from build123d import *

# Parameters (mm, degrees)
SKETCH1_W                 = 113.5
SKETCH1_H                 = 8.5
BOSS_EXTRUDE1_DEPTH       = 8.5
BOSS_EXTRUDE2_DEPTH       = 5
BOSS_EXTRUDE3_DEPTH       = 5
SKETCH13_W                = 91.5
SKETCH13_H                = 6.5
CUT_EXTRUDE1_DEPTH        = 6.5
M3X0_5_TAPPED_HOLE1_D     = 2.5
M3X0_5_TAPPED_HOLE1_DEPTH = 7.5
M3X0_5_TAPPED_HOLE1_TIP   = 0.751075774
M3X0_5_TAPPED_HOLE2_D     = 2.5
M3X0_5_TAPPED_HOLE2_DEPTH = 5
M3X0_5_TAPPED_HOLE3_D     = 2.5
M3X0_5_TAPPED_HOLE3_DEPTH = 5
M3X0_5_TAPPED_HOLE4_D     = 2.5
M3X0_5_TAPPED_HOLE4_DEPTH = 7.5
M3X0_5_TAPPED_HOLE4_TIP   = 0.751075774
FILLET1_R                 = 1
FILLET2_R                 = 1
FILLET3_R                 = 1
FILLET4_R                 = 3
M3X0_5_TAPPED_HOLE5_D     = 2.5
M3X0_5_TAPPED_HOLE5_DEPTH = 7.5
M3X0_5_TAPPED_HOLE5_TIP   = 0.751075774
M3X0_5_TAPPED_HOLE6_D     = 2.5
M3X0_5_TAPPED_HOLE6_DEPTH = 7.5
M3X0_5_TAPPED_HOLE6_TIP   = 0.751075774
M3X0_5_TAPPED_HOLE7_D     = 2.5
M3X0_5_TAPPED_HOLE7_DEPTH = 7.5
M3X0_5_TAPPED_HOLE7_TIP   = 0.751075774
M3X0_5_TAPPED_HOLE9_D     = 2.5
M3X0_5_TAPPED_HOLE9_DEPTH = 7.5
M3X0_5_TAPPED_HOLE9_TIP   = 0.751075774
SKETCH43_W                = 10.5
SKETCH43_H                = 10.5
CUT_EXTRUDE3_DEPTH        = 110.01404726
SKETCH44_R                = 2.5
CUT_EXTRUDE4_DEPTH        = 10
CUT_EXTRUDE5_REACH        = 107.072
SKETCH45_R                = 1.25
M6_TAPPED_HOLE1_D         = 5
M6_TAPPED_HOLE1_DEPTH     = 3.05
M6_TAPPED_HOLE1_TIP       = 1.502151548


with BuildPart() as part:
    # Sketch1 → Boss-Extrude1 (new body)
    with BuildSketch(Plane.XY):
        Rectangle(SKETCH1_W, SKETCH1_H)
    extrude(amount=BOSS_EXTRUDE1_DEPTH)

    # Sketch4 → Boss-Extrude2 (add)
    with BuildSketch(Plane(origin=(50.75, 0, 0), x_dir=(0, 0, -1), z_dir=(1, 0, 0))):
        Polygon((0, -2.25), (10.5, -2.25), (10.5, 14.75), (-6.5, 14.75), (-6.5, 4.25), (0, 4.25), align=None)
    extrude(amount=-BOSS_EXTRUDE2_DEPTH)

    # Sketch12 → Boss-Extrude3 (add)
    with BuildSketch(Plane.ZY.offset(50.75)):
        Polygon((6.5, 4.25), (6.5, 14.75), (-10.5, 14.75), (-10.5, -2.25), (0, -2.25), (0, 4.25), align=None)
    extrude(amount=-BOSS_EXTRUDE3_DEPTH)

    # Sketch13 → Cut-Extrude1 (cut)
    with BuildSketch(Plane(origin=(0, 4.25, 0), x_dir=(1, 0, 0), z_dir=(0, 1, 0))):
        with Locations((0, -3.25)):
            Rectangle(SKETCH13_W, SKETCH13_H)
    extrude(amount=-CUT_EXTRUDE1_DEPTH, mode=Mode.SUBTRACT)

    # M3x0.5 Tapped Hole1
    with Locations(Plane.XY.offset(6.5)):
        with Locations((-48.25, 7.75)):
            Hole(M3X0_5_TAPPED_HOLE1_D / 2, depth=M3X0_5_TAPPED_HOLE1_DEPTH)
            with Locations((0, 0, -(M3X0_5_TAPPED_HOLE1_DEPTH + M3X0_5_TAPPED_HOLE1_TIP / 2))):  # 118° drill point
                Cone(0, M3X0_5_TAPPED_HOLE1_D / 2, M3X0_5_TAPPED_HOLE1_TIP, mode=Mode.SUBTRACT)

    # M3x0.5 Tapped Hole2
    with Locations(Plane.ZY.offset(50.75)):
        with Locations((3.25, 12.25)):
            Hole(M3X0_5_TAPPED_HOLE2_D / 2, depth=M3X0_5_TAPPED_HOLE2_DEPTH)

    # M3x0.5 Tapped Hole3
    with Locations(Plane.ZY.offset(50.75)):
        with Locations((-8, 1)):
            Hole(M3X0_5_TAPPED_HOLE3_D / 2, depth=M3X0_5_TAPPED_HOLE3_DEPTH)

    # M3x0.5 Tapped Hole4
    with Locations(Plane.XZ.offset(2.25)):
        with Locations((-48.25, -3.5)):
            Hole(M3X0_5_TAPPED_HOLE4_D / 2, depth=M3X0_5_TAPPED_HOLE4_DEPTH)
            with Locations((0, 0, -(M3X0_5_TAPPED_HOLE4_DEPTH + M3X0_5_TAPPED_HOLE4_TIP / 2))):  # 118° drill point
                Cone(0, M3X0_5_TAPPED_HOLE4_D / 2, M3X0_5_TAPPED_HOLE4_TIP, mode=Mode.SUBTRACT)

    # Fillet1
    fillet1_edges = [part.edges().sort_by_distance(p)[0] for p in [
        (0, -4.25, 8.5),
    ]]
    fillet(fillet1_edges, radius=FILLET1_R)

    # Fillet2
    fillet2_edges = [part.edges().sort_by_distance(p)[0] for p in [
        (-56.75, 0.5, 8.5),
        (-56.75, 0, 0),
        (-56.75, 4.25, 4.25),
        (-56.75, -4.25, 3.75),
        (-56.75, -3.957106781, 8.207106781),
    ]]
    fillet(fillet2_edges, radius=FILLET2_R)

    # Fillet3
    fillet3_edges = [part.edges().sort_by_distance(p)[0] for p in [
        (56.75, 0, 0),
        (56.75, 4.25, 4.25),
        (56.75, 0.5, 8.5),
        (56.75, -4.25, 3.75),
        (56.75, -3.957106781, 8.207106781),
    ]]
    fillet(fillet3_edges, radius=FILLET3_R)

    # Fillet4
    fillet4_edges = [part.edges().sort_by_distance(p)[0] for p in [
        (-45.75, 1, 6.5),
        (45.75, 1, 6.5),
    ]]
    fillet(fillet4_edges, radius=FILLET4_R)

    # M3x0.5 Tapped Hole5
    with Locations(Plane.XY.offset(6.5)):
        with Locations((48.25, 7.75)):
            Hole(M3X0_5_TAPPED_HOLE5_D / 2, depth=M3X0_5_TAPPED_HOLE5_DEPTH)
            with Locations((0, 0, -(M3X0_5_TAPPED_HOLE5_DEPTH + M3X0_5_TAPPED_HOLE5_TIP / 2))):  # 118° drill point
                Cone(0, M3X0_5_TAPPED_HOLE5_D / 2, M3X0_5_TAPPED_HOLE5_TIP, mode=Mode.SUBTRACT)

    # M3x0.5 Tapped Hole6
    with Locations(Plane.XZ.offset(2.25)):
        with Locations((48.25, -3.5)):
            Hole(M3X0_5_TAPPED_HOLE6_D / 2, depth=M3X0_5_TAPPED_HOLE6_DEPTH)
            with Locations((0, 0, -(M3X0_5_TAPPED_HOLE6_DEPTH + M3X0_5_TAPPED_HOLE6_TIP / 2))):  # 118° drill point
                Cone(0, M3X0_5_TAPPED_HOLE6_D / 2, M3X0_5_TAPPED_HOLE6_TIP, mode=Mode.SUBTRACT)

    # M3x0.5 Tapped Hole7
    with Locations(Plane(origin=(50.75, 0, 0), x_dir=(0, 0, -1), z_dir=(1, 0, 0))):
        with Locations((8, 1)):
            Hole(M3X0_5_TAPPED_HOLE7_D / 2, depth=M3X0_5_TAPPED_HOLE7_DEPTH)
            with Locations((0, 0, -(M3X0_5_TAPPED_HOLE7_DEPTH + M3X0_5_TAPPED_HOLE7_TIP / 2))):  # 118° drill point
                Cone(0, M3X0_5_TAPPED_HOLE7_D / 2, M3X0_5_TAPPED_HOLE7_TIP, mode=Mode.SUBTRACT)

    # M3x0.5 Tapped Hole9
    with Locations(Plane(origin=(50.75, 0, 0), x_dir=(0, 0, -1), z_dir=(1, 0, 0))):
        with Locations((-3.25, 12.25)):
            Hole(M3X0_5_TAPPED_HOLE9_D / 2, depth=M3X0_5_TAPPED_HOLE9_DEPTH)
            with Locations((0, 0, -(M3X0_5_TAPPED_HOLE9_DEPTH + M3X0_5_TAPPED_HOLE9_TIP / 2))):  # 118° drill point
                Cone(0, M3X0_5_TAPPED_HOLE9_D / 2, M3X0_5_TAPPED_HOLE9_TIP, mode=Mode.SUBTRACT)

    # Sketch43 → Cut-Extrude3 (cut, through all)
    with BuildSketch(Plane.ZY.offset(50.75)):
        with Locations((-5.25, 9.5)):
            Rectangle(SKETCH43_W, SKETCH43_H)
    extrude(amount=-CUT_EXTRUDE3_DEPTH, mode=Mode.SUBTRACT)

    # Sketch44 → Cut-Extrude4 (cut)
    with BuildSketch(Plane(origin=(56.75, 0, 0), x_dir=(0, 0, -1), z_dir=(1, 0, 0))):
        with Locations((-4.25, 0)):
            Circle(SKETCH44_R)
    extrude(amount=-CUT_EXTRUDE4_DEPTH, mode=Mode.SUBTRACT)

    # Sketch45 → Cut-Extrude5 (cut, up to next)
    with BuildSketch(Plane(origin=(46.75, 0, 0), x_dir=(0, 0, -1), z_dir=(1, 0, 0)), mode=Mode.PRIVATE) as cut_extrude5_sk1:
        with Locations((-4.25, 0)):
            Circle(SKETCH45_R)
    cut_extrude5_tool1 = extrude(cut_extrude5_sk1.sketch, amount=-CUT_EXTRUDE5_REACH, mode=Mode.PRIVATE) & part.part
    add(cut_extrude5_tool1.solids().sort_by_distance((46.75, 0, 4.25))[0], mode=Mode.SUBTRACT)

    # M6 Tapped Hole1
    with Locations(Plane(origin=(56.75, 0, 0), x_dir=(0, 0, -1), z_dir=(1, 0, 0))):
        with Locations((-4.25, 0)):
            Hole(M6_TAPPED_HOLE1_D / 2, depth=M6_TAPPED_HOLE1_DEPTH)
            with Locations((0, 0, -(M6_TAPPED_HOLE1_DEPTH + M6_TAPPED_HOLE1_TIP / 2))):  # 118° drill point
                Cone(0, M6_TAPPED_HOLE1_D / 2, M6_TAPPED_HOLE1_TIP, mode=Mode.SUBTRACT)


solid = part.part
Can you work these out from the model? Positions are in its coordinate system, mm. A direction names the side the tool comes from. Round coordinates to 2 decimals unless told otherwise and drop trailing zeros. Order: outer loops, then holes, each group sorted by start corner. A loop starts at its lowest first (then second) coordinate and runs counter-clockwise, first axis right, second up. Notation, with made-up numbers: (-16.75, 81.5) - (17.25, 81.5) arc R14 ccw to (17.25, 88.5) - close; hole circle Ø9 at (65, -39). An arc over 180 degrees is marked (long way). Answer in a Markdown table with one row per item.
(1) Please list where these lines run through material, in increasing order: L1, parallel to X at y = 3.25, z = -1.5; L2, parallel to Y at x = -42, z = 2.75; L3, parallel to Y at x = 46, z = 4.25. Write a range as from..to.
From the geometry:
| item | result |
|---|---|
| L1 | x = -50.75..-45.75, 45.75..50.75 |
| L2 | y = -4.25..-2.25 |
| L3 | y = -4.25..-1.25, 1.25..11.5, 13..14.75 |
(2) Suppose I cut it at B-B, the plane z = -8. Please give me the cut outline in (x, y), plus the area to 3 significant figures.
From the geometry:
| item | result |
|---|---|
| outline | (-50.75, -2.25) - (-45.75, -2.25) - (-45.75, -0.25) - (-50.75, -0.25) - close; (-50.75, 2.25) - (-45.75, 2.25) - (-45.75, 4.25) - (-50.75, 4.25) - close; (45.75, -2.25) - (50.75, -2.25) - (50.75, -0.25) - (45.75, -0.25) - close; (45.75, 2.25) - (50.75, 2.25) - (50.75, 4.25) - (45.75, 4.25) - close |
| area | 40.0 mm2 |
(3) If we mould it in two halves opening along Z, with no side actions, what happens to faces 1 (the face through (-0.3, -2.5, 0)), 2 (the face through (-45.75, 3, 0)), 3 (the face through (-48.215, 13.304, 2.578))? For each: released by +Z, released by -Z, zero draft, split by the parting line, or undercut.
From the geometry:
| item | result |
|---|---|
| face 1 | released by -Z |
| face 2 | zero draft |
| face 3 | undercut |
(4) Suppose I cut it at A-A, the plane x = 48.25. Please give me the cut outline in (y, z).
From the geometry:
| item | result |
|---|---|
| outline | (-4.25, 0) - (-2.25, 0) - (-2.25, -2.25) - (4.25, -2.25) - (4.25, 0) - (6.5, 0) - (6.5, 6.5) - (4.25, 6.5) - (4.25, 8.5) - (-3.25, 8.5) arc R1 ccw to (-4.25, 7.5) - close; (-2.25, -10.5) - (4.25, -10.5) - (4.25, -4.75) - (-2.25, -4.75) - close; (9, 0) - (14.75, 0) - (14.75, 6.5) - (9, 6.5) - close; hole circle Ø5 at (0, 4.25); hole circle Ø2.5 at (1, -8); hole circle Ø2.5 at (12.25, 3.25) |
(5) Which directions (+Z, -Z, +X, -X, +Y, -Y) give clear straight access to the entire face, cutting with the end or side of a thin tool? Please do faces 4 (the face through (50.75, 10, 3)), 5 (the face through (51.82, 0.751, 1.865)), 6 (the face through (-1, 1, 6.5)), 7 (the face through (-48, 4.25, -5)), 8 (the face through (48, -2.25, -5)).
From the geometry:
| item | result |
|---|---|
| face 4 | +Z, -Z, +X, +Y |
| face 5 | +X |
| face 6 | -Z, +Y |
| face 7 | -Z, +X, -X, +Y |
| face 8 | -Z, +X, -X, -Y |
(6) Suppose I cut it at C-C, the plane x = -13. Please give me the cut outline in (y, z), plus the area to 3 significant figures.
From the geometry:
| item | result |
|---|---|
| outline | (-4.25, 0) - (-2.25, 0) - (-2.25, 6.5) - (4.25, 6.5) - (4.25, 8.5) - (-3.25, 8.5) arc R1 ccw to (-4.25, 7.5) - close |
| area | 29.8 mm2 |
(7) Suppose I cut it at D-D, the plane z = -3.5. Please give me the cut outline in (x, y).
From the geometry:
| item | result |
|---|---|
| outline | (-50.75, -2.25) - (-49.5, -2.25) - (-49.5, 4.25) - (-50.75, 4.25) - close; (-47, -2.25) - (-45.75, -2.25) - (-45.75, 4.25) - (-47, 4.25) - close; (45.75, -2.25) - (47, -2.25) - (47, 4.25) - (45.75, 4.25) - close; (49.5, -2.25) - (50.75, -2.25) - (50.75, 4.25) - (49.5, 4.25) - close |
(8) For P1, Ø10, axis at y = -2, z = 0, coming from the -X side; P2, Ø1.5, axis at y = 7.5, z = 3.5, coming from the +X side; P3, Ø2.5, axis at x = -12, y = 2, coming from the -Z side; P4, Ø4, axis at x = -47.5, y = 7.5, coming from the +Z side, each with a flat end and sliding along its axis, tell me the tip position at first contact or that it passes through.
From the geometry:
| item | result |
|---|---|
| P1 | stops at x = -56.75 |
| P2 | stops at x = 50.75 |
| P3 | stops at z = 6.5 |
| P4 | stops at z = 6.5 |
